Can you work these out from the drawing? Everything is in mm from the part's minimum corner. Give positions to 0.01 mm unless a question says otherwise; leave off trailing zeros. Order: outer loops, then holes, each group sorted by start corner. A loop starts at its lowest first (then second) coordinate and runs counter-clockwise, first axis right, second up. Notation, with made-up numbers: (58.5, 69) - (79.5, 69) arc R14 cw to (79.5, 85) - close; hole circle Ø2 at (49, -5.5). An arc over 180 degrees is marked (long way). One line per question, with ' | ' between items.
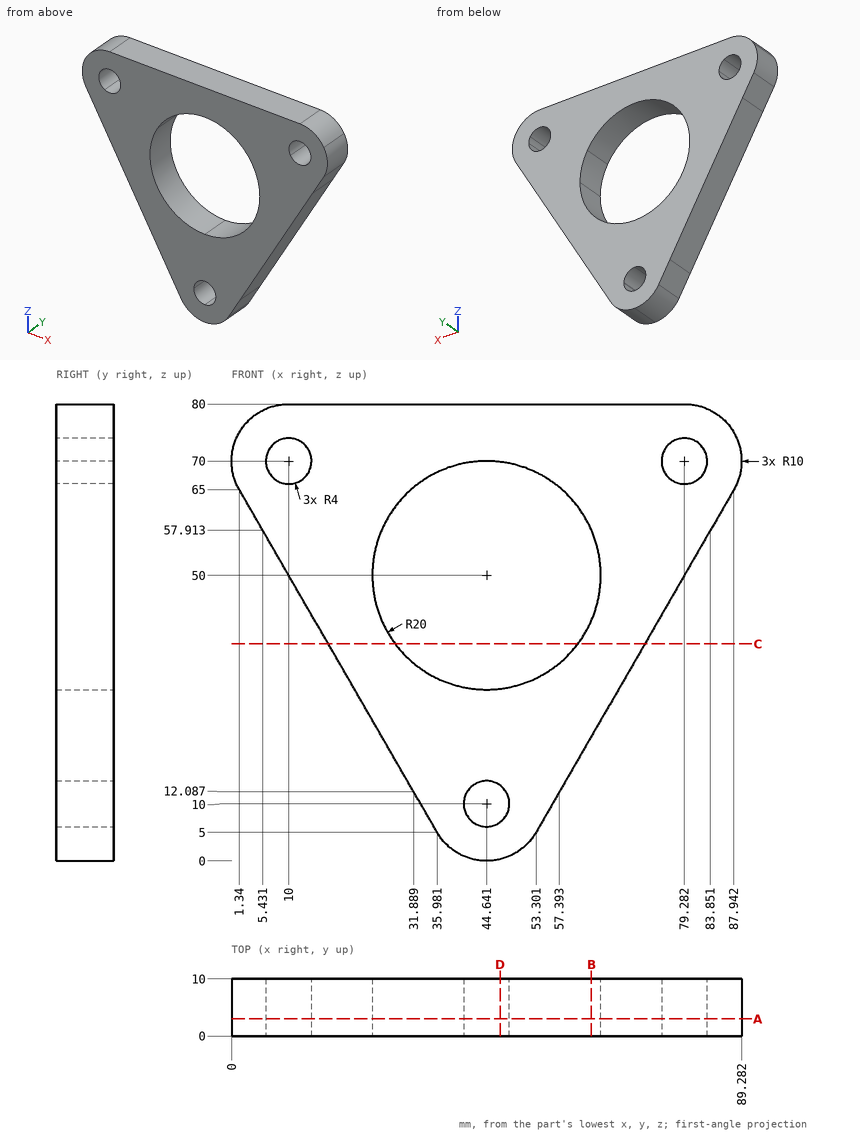
(1) Imagine slicing it at A-A (y = 3). Count the separate pieces of the cut face and the enclosed holes in it, and give its area (3 significant figures).
Answer below:
separate pieces: 1 | enclosed holes: 4 | area: 3,060 mm^2
(2) Imagine slicing it at C-C (z = 38). List the corners of the cut face in (x, y) for me.
Answer below:
outline: (16.93, 0) - (28.64, 0) - (28.64, 10) - (16.93, 10) - close; (60.64, 0) - (72.35, 0) - (72.35, 10) - (60.64, 10) - close
(3) Imagine slicing it at D-D (x = 47). List the corners of the cut face in (y, z) for me, and give its area (3 significant figures).
Answer below:
outline: (0, 0.28) - (10, 0.28) - (10, 6.77) - (0, 6.77) - close; (0, 13.23) - (10, 13.23) - (10, 30.14) - (0, 30.14) - close; (0, 69.86) - (10, 69.86) - (10, 80) - (0, 80) - close | area: 335 mm^2
(4) If I drill on line 1 (Z direction, x = 45, y = 9.25) (1 decimal); line 2 (Z direction, x = 52, y = 6.25) (1 decimal); line 3 (Z direction, x = 41, y = 7.5) (1 decimal), over which ranges is the centre line in solid material (lowest first)?
Answer below:
line 1: 0 to 6, 14 to 30, 70 to 80 | line 2: 3.2 to 31.4, 68.6 to 80 | line 3: 0.7 to 8.3, 11.7 to 30.3, 69.7 to 80
(5) Imagine slicing it at B-B (x = 63). List the corners of the cut face in (y, z) for me, and give its area (3 significant figures).
Answer below:
outline: (0, 21.8) - (10, 21.8) - (10, 42.07) - (0, 42.07) - close; (0, 57.93) - (10, 57.93) - (10, 80) - (0, 80) - close | area: 423 mm^2
(6) Will these pins go through, and if not, where does the flat tip stop? pin 1 (5 mm diameter, centred on x = 77, y = 7.5, fed in from -Z) (1 decimal); pin 2 (6 mm diameter, centred on y = 7, z = 43.5, fed in from +X); pin 3 (5 mm diameter, centred on x = 73, y = 2, fed in from -Z).
Answer below:
pin 1: z = 41.7 | pin 2: x = 77.26 | pin 3: z = 34.79
